```python
from build123d import *

# Parameters (mm, degrees)
BOSS_EXTRUDE1_DEPTH = 10
SKETCH3_R           = 4
CUT_EXTRUDE1_DEPTH  = 4
SKETCH4_R           = 2.5
CUT_EXTRUDE2_DEPTH  = 10


with BuildPart() as part:
    # Sketch2 → Boss-Extrude1 (new body)
    with BuildSketch(Plane.XY):
        with BuildLine():
            Line((2.133108761, 10.808181691), (2.19765063, 11.135206855))
            ThreePointArc((2.19765063, 11.135206855), (0, 11.35), (-2.19765063, 11.135206855))
            Line((-2.19765063, 11.135206855), (-2.133108761, 10.808181691))
            ThreePointArc((-2.133108761, 10.808181691), (-1.817325769, 10.865738424), (-1.5, 10.914070939))
            Line((-1.5, 10.914070939), (-1.5, 5.598076211))
            Line((-1.5, 5.598076211), (-4.157997364, 10.201862691))
            ThreePointArc((-4.157997364, 10.201862691), (-3.859018929, 10.318668391), (-3.556764469, 10.426714294))
            Line((-3.556764469, 10.426714294), (-3.664382154, 10.742197328))
            ThreePointArc((-3.664382154, 10.742197328), (-5.675, 9.829388333), (-7.470824702, 8.544546698))
            Line((-7.470824702, 8.544546698), (-7.251417222, 8.293605533))
            ThreePointArc((-7.251417222, 8.293605533), (-7.006719495, 8.501342622), (-6.756073575, 8.701862691))
            Line((-6.756073575, 8.701862691), (-4.098076211, 4.098076211))
            Line((-4.098076211, 4.098076211), (-8.701862691, 6.756073575))
            ThreePointArc((-8.701862691, 6.756073575), (-8.501342622, 7.006719495), (-8.293605533, 7.251417222))
            Line((-8.293605533, 7.251417222), (-8.544546698, 7.470824702))
            ThreePointArc((-8.544546698, 7.470824702), (-9.829388333, 5.675), (-10.742197328, 3.664382154))
            Line((-10.742197328, 3.664382154), (-10.426714294, 3.556764469))
            ThreePointArc((-10.426714294, 3.556764469), (-10.318668391, 3.859018929), (-10.201862691, 4.157997364))
            Line((-10.201862691, 4.157997364), (-5.598076211, 1.5))
            Line((-5.598076211, 1.5), (-10.914070939, 1.5))
            ThreePointArc((-10.914070939, 1.5), (-10.865738424, 1.817325769), (-10.808181691, 2.133108761))
            Line((-10.808181691, 2.133108761), (-11.135206855, 2.19765063))
            ThreePointArc((-11.135206855, 2.19765063), (-11.35, 0), (-11.135206855, -2.19765063))
            Line((-11.135206855, -2.19765063), (-10.808181691, -2.133108761))
            ThreePointArc((-10.808181691, -2.133108761), (-10.865738424, -1.817325769), (-10.914070939, -1.5))
            Line((-10.914070939, -1.5), (-5.598076211, -1.5))
            Line((-5.598076211, -1.5), (-10.201862691, -4.157997364))
            ThreePointArc((-10.201862691, -4.157997364), (-10.318668391, -3.859018929), (-10.426714294, -3.556764469))
            Line((-10.426714294, -3.556764469), (-10.742197328, -3.664382154))
            ThreePointArc((-10.742197328, -3.664382154), (-9.829388333, -5.675), (-8.544546698, -7.470824702))
            Line((-8.544546698, -7.470824702), (-8.293605533, -7.251417222))
            ThreePointArc((-8.293605533, -7.251417222), (-8.501342622, -7.006719495), (-8.701862691, -6.756073575))
            Line((-8.701862691, -6.756073575), (-4.098076211, -4.098076211))
            Line((-4.098076211, -4.098076211), (-6.756073575, -8.701862691))
            ThreePointArc((-6.756073575, -8.701862691), (-7.006719495, -8.501342622), (-7.251417222, -8.293605533))
            Line((-7.251417222, -8.293605533), (-7.470824702, -8.544546698))
            ThreePointArc((-7.470824702, -8.544546698), (-5.675, -9.829388333), (-3.664382154, -10.742197328))
            Line((-3.664382154, -10.742197328), (-3.556764469, -10.426714294))
            ThreePointArc((-3.556764469, -10.426714294), (-3.859018929, -10.318668391), (-4.157997364, -10.201862691))
            Line((-4.157997364, -10.201862691), (-1.5, -5.598076211))
            Line((-1.5, -5.598076211), (-1.5, -10.914070939))
            ThreePointArc((-1.5, -10.914070939), (-1.817325769, -10.865738424), (-2.133108761, -10.808181691))
            Line((-2.133108761, -10.808181691), (-2.19765063, -11.135206855))
            ThreePointArc((-2.19765063, -11.135206855), (0, -11.35), (2.19765063, -11.135206855))
            Line((2.19765063, -11.135206855), (2.133108761, -10.808181691))
            ThreePointArc((2.133108761, -10.808181691), (1.817325769, -10.865738424), (1.5, -10.914070939))
            Line((1.5, -10.914070939), (1.5, -5.598076211))
            Line((1.5, -5.598076211), (4.157997364, -10.201862691))
            ThreePointArc((4.157997364, -10.201862691), (3.859018929, -10.318668391), (3.556764469, -10.426714294))
            Line((3.556764469, -10.426714294), (3.664382154, -10.742197328))
            ThreePointArc((3.664382154, -10.742197328), (5.675, -9.829388333), (7.470824702, -8.544546698))
            Line((7.470824702, -8.544546698), (7.251417222, -8.293605533))
            ThreePointArc((7.251417222, -8.293605533), (7.006719495, -8.501342622), (6.756073575, -8.701862691))
            Line((6.756073575, -8.701862691), (4.098076211, -4.098076211))
            Line((4.098076211, -4.098076211), (8.701862691, -6.756073575))
            ThreePointArc((8.701862691, -6.756073575), (8.501342622, -7.006719495), (8.293605533, -7.251417222))
            Line((8.293605533, -7.251417222), (8.544546698, -7.470824702))
            ThreePointArc((8.544546698, -7.470824702), (9.829388333, -5.675), (10.742197328, -3.664382154))
            Line((10.742197328, -3.664382154), (10.426714294, -3.556764469))
            ThreePointArc((10.426714294, -3.556764469), (10.318668391, -3.859018929), (10.201862691, -4.157997364))
            Line((10.201862691, -4.157997364), (5.598076211, -1.5))
            Line((5.598076211, -1.5), (10.914070939, -1.5))
            ThreePointArc((10.914070939, -1.5), (10.865738424, -1.817325769), (10.808181691, -2.133108761))
            Line((10.808181691, -2.133108761), (11.135206855, -2.19765063))
            ThreePointArc((11.135206855, -2.19765063), (11.35, 0), (11.135206855, 2.19765063))
            Line((11.135206855, 2.19765063), (10.808181691, 2.133108761))
            ThreePointArc((10.808181691, 2.133108761), (10.865738424, 1.817325769), (10.914070939, 1.5))
            Line((10.914070939, 1.5), (5.598076211, 1.5))
            Line((5.598076211, 1.5), (10.201862691, 4.157997364))
            ThreePointArc((10.201862691, 4.157997364), (10.318668391, 3.859018929), (10.426714294, 3.556764469))
            Line((10.426714294, 3.556764469), (10.742197328, 3.664382154))
            ThreePointArc((10.742197328, 3.664382154), (9.829388333, 5.675), (8.544546698, 7.470824702))
            Line((8.544546698, 7.470824702), (8.293605533, 7.251417222))
            ThreePointArc((8.293605533, 7.251417222), (8.501342622, 7.006719495), (8.701862691, 6.756073575))
            Line((8.701862691, 6.756073575), (4.098076211, 4.098076211))
            Line((4.098076211, 4.098076211), (6.756073575, 8.701862691))
            ThreePointArc((6.756073575, 8.701862691), (7.006719495, 8.501342622), (7.251417222, 8.293605533))
            Line((7.251417222, 8.293605533), (7.470824702, 8.544546698))
            ThreePointArc((7.470824702, 8.544546698), (5.675, 9.829388333), (3.664382154, 10.742197328))
            Line((3.664382154, 10.742197328), (3.556764469, 10.426714294))
            ThreePointArc((3.556764469, 10.426714294), (3.859018929, 10.318668391), (4.157997364, 10.201862691))
            Line((4.157997364, 10.201862691), (1.5, 5.598076211))
            Line((1.5, 5.598076211), (1.5, 10.914070939))
            ThreePointArc((1.5, 10.914070939), (1.817325769, 10.865738424), (2.133108761, 10.808181691))
        make_face()
    extrude(amount=BOSS_EXTRUDE1_DEPTH)

    # Sketch3 → Cut-Extrude1 (cut)
    with BuildSketch(Plane.XY.offset(10)):
        Circle(SKETCH3_R)
    extrude(amount=-CUT_EXTRUDE1_DEPTH, mode=Mode.SUBTRACT)

    # Sketch4 → Cut-Extrude2 (cut)
    with BuildSketch(Plane.XY.offset(6)):
        Circle(SKETCH4_R)
    extrude(amount=-CUT_EXTRUDE2_DEPTH, mode=Mode.SUBTRACT)


solid = part.part
```
Input: part model. Units: mm. Frame: model coordinates. A direction names the side the tool comes from. Round coordinates to 2 decimals unless told otherwise and drop trailing zeros. Loops run counter-clockwise (first coordinate to the right, second up) from the corner with the lowest first, then second, coordinate; pieces in that order, holes last.
1) Set-up query: faces 1 (the cylindrical face through (-9.845, -5.648, 4.93)), 2 (the flat face through (8, -1.5, 5)). Return all of +Z, -Z, +X, -X, +Y, -Y with unobstructed straight access to the full face (end or side cutting, diameter ignored); none if empty.
Ans:
face 1: +Z, -Z, -X, -Y
face 2: +Z, -Z
2) Pin query (flat end, axial travel): pin 1 (6 mm diameter, centred on y = -7, z = 3.5, fed in from +X); pin 2 (4 mm diameter, centred on x = 0.5, y = 1.5, fed in from +Z); pin 3 (2.5 mm diameter, centred on x = 9, z = 4, fed in from -Y). Return the tip coordinate at first contact, or that it passes through.
Ans:
pin 1: stops at x = 10.62
pin 2: stops at z = 6
pin 3: stops at y = -7.47
3) Material intervals for line 1 (Y direction, x = 0, z = 7.6); line 2 (Y direction, x = 0, z = 2.65); line 3 (X direction, y = 7, z = 7.75), sorted ascending.
Ans:
line 1: y = -11.35 to -4, 4 to 11.35
line 2: y = -11.35 to -2.5, 2.5 to 11.35
line 3: x = -8.93 to -8.51, -5.77 to -2.31, -1.5 to 1.5, 2.31 to 5.77, 8.51 to 8.93
4) Section query C-C on x = 0. Return the cut outline in (y, z).
Ans:
outline: (-11.35, 0) - (-2.5, 0) - (-2.5, 6) - (-4, 6) - (-4, 10) - (-11.35, 10) - close; (2.5, 0) - (11.35, 0) - (11.35, 10) - (4, 10) - (4, 6) - (2.5, 6) - close
5) Section query B-B on y = 1. Return the cut outline in (x, z).
Ans:
outline: (-11.31, 0) - (-2.29, 0) - (-2.29, 6) - (-3.87, 6) - (-3.87, 10) - (-11.31, 10) - close; (2.29, 0) - (11.31, 0) - (11.31, 10) - (3.87, 10) - (3.87, 6) - (2.29, 6) - close
6) Section query D-D on y = 8. Return the cut outline in (x, z).
Ans:
outline: (-6.35, 0) - (-2.89, 0) - (-2.89, 10) - (-6.35, 10) - close; (-1.5, 0) - (1.5, 0) - (1.5, 10) - (-1.5, 10) - close; (2.89, 0) - (6.35, 0) - (6.35, 10) - (2.89, 10) - close
7) Pull-direction query (Y, two-part tool) for faces 3 (the cylindrical face through (5.702, 9.814, 4.93)), 4 (the cylindrical face through (5.648, -9.845, 4.93)), 5 (the flat face through (2, -2, 0)), 6 (the flat face through (-6.37, 5.41, 4.93)); classes: released by +Y, released by -Y, zero draft, split by the parting line, or undercut.
Ans:
face 3: released by +Y
face 4: released by -Y
face 5: zero draft
face 6: undercut
8) Section query A-A on x = -9.5. Return the cut outline in (y, z), plus the area to 3 significant figures.
Ans:
outline: (-6.21, 0) - (-3.75, 0) - (-3.75, 10) - (-6.21, 10) - close; (-1.5, 0) - (1.5, 0) - (1.5, 10) - (-1.5, 10) - close; (3.75, 0) - (6.21, 0) - (6.21, 10) - (3.75, 10) - close
area: 79.2 mm2
